The model under review builds one solid part; all positions refer to its coordinate system, in mm. A direction names the side the tool comes from. Coordinates: 2 decimals unless noted, no trailing zeros. Write each loop counter-clockwise with the first axis right and the second up, starting at its lowest first coordinate (ties: lowest second). Pieces come first, ordered by that corner, then holes. Notation, with made-up numbers: (49, 63.25) - (80, 63.25) arc R20 ccw to (80, 90.25) - close; hole circle Ø4 at (-35, -13). An arc over 180 degrees is marked (long way). Put each result on its own line as item: value.
from build123d import *

# Parameters (mm, degrees)
CROQUIS1_W              = 45.4
CROQUIS1_H              = 20.4
SALIENTE_EXTRUIR1_DEPTH = 1.6
CROQUIS2_R              = 0.7
CORTAR_EXTRUIR1_DEPTH   = 1
SALIENTE_EXTRUIR2_DEPTH = 0.5
SALIENTE_EXTRUIR3_DEPTH = 3
CROQUIS9_R              = 7.95
SALIENTE_EXTRUIR4_DEPTH = 11
CROQUIS10_W             = 10
CROQUIS10_H             = 1
SALIENTE_EXTRUIR5_DEPTH = 2
CROQUIS12_W             = 0.5
CROQUIS12_H             = 0.5
REDONDEO4_R             = 0.7
MATRIZL1_COUNT          = 4
MATRIZL1_PITCH          = 2.5
REDONDEO5_R             = 1
CROQUIS13_W             = 9
CROQUIS13_H             = 3
SALIENTE_EXTRUIR6_DEPTH = 1.5
MATRIZL2_COUNT          = 2
MATRIZL2_PITCH          = 18
CROQUIS14_W             = 3
CROQUIS14_H             = 9
SALIENTE_EXTRUIR7_DEPTH = 1.5
REDONDEO6_R             = 0.7


with BuildPart() as part:
    # Croquis1 → Saliente-Extruir1 (new body)
    with BuildSketch(Plane(origin=(0, 0, 0), x_dir=(1, 0, 0), z_dir=(0, 1, 0))):
        Rectangle(CROQUIS1_W, CROQUIS1_H)
    extrude(amount=SALIENTE_EXTRUIR1_DEPTH)

    # Croquis2 → Cortar-Extruir1 (cut)
    with BuildSketch(Plane(origin=(0, 1.6, 0), x_dir=(1, 0, 0), z_dir=(0, 1, 0))):
        with Locations((-21.5, 9)):
            Circle(CROQUIS2_R)
        with Locations((21.5, 9)):
            Circle(CROQUIS2_R)
        with Locations((21.5, -9)):
            Circle(CROQUIS2_R)
        with Locations((-21.5, -9)):
            Circle(CROQUIS2_R)
    extrude(amount=-CORTAR_EXTRUIR1_DEPTH, mode=Mode.SUBTRACT)

    # Croquis3 → Saliente-Extruir2 (add)
    with BuildSketch(Plane(origin=(0, 1.6, 0), x_dir=(1, 0, 0), z_dir=(0, 1, 0))):
        with BuildLine():
            Line((-4.202221616, 9.535810589), (4.202221616, 9.535810589))
            ThreePointArc((4.202221616, 9.535810589), (5.818460699, 7.919571506), (4.202221616, 6.303332424))
            Line((4.202221616, 6.303332424), (-4.202221616, 6.303332424))
            ThreePointArc((-4.202221616, 6.303332424), (-5.818460699, 7.919571506), (-4.202221616, 9.535810589))
        make_face()
        with BuildLine():
            Line((-4.202221616, 9.304919292), (4.202221616, 9.304919292))
            ThreePointArc((4.202221616, 9.304919292), (5.587569401, 7.919571506), (4.202221616, 6.534223721))
            Line((4.202221616, 6.534223721), (-4.202221616, 6.534223721))
            ThreePointArc((-4.202221616, 6.534223721), (-5.587569401, 7.919571506), (-4.202221616, 9.304919292))
        make_face(mode=Mode.SUBTRACT)
    extrude(amount=SALIENTE_EXTRUIR2_DEPTH)

    # Croquis8 → Saliente-Extruir3 (add)
    with BuildSketch(Plane(origin=(0, 1.6, 0), x_dir=(1, 0, 0), z_dir=(0, 1, 0))):
        with BuildLine():
            Line((-4.202221616, 9.304919292), (4.202221616, 9.304919292))
            ThreePointArc((4.202221616, 9.304919292), (5.587569401, 7.919571506), (4.202221616, 6.534223721))
            Line((4.202221616, 6.534223721), (-4.202221616, 6.534223721))
            ThreePointArc((-4.202221616, 6.534223721), (-5.587569401, 7.919571506), (-4.202221616, 9.304919292))
        make_face()
    extrude(amount=SALIENTE_EXTRUIR3_DEPTH)

    # Croquis9 → Saliente-Extruir4 (add)
    with BuildSketch(Plane(origin=(0, 1.6, 0), x_dir=(1, 0, 0), z_dir=(0, 1, 0))):
        with Locations((-13.1, 0)):
            Circle(CROQUIS9_R)
        with Locations((13.1, 0)):
            Circle(CROQUIS9_R)
    extrude(amount=SALIENTE_EXTRUIR4_DEPTH)

    # Croquis10 → Saliente-Extruir5 (add)
    with BuildSketch(Plane.XZ):
        with Locations((-0.012747973, 9.7)):
            Rectangle(CROQUIS10_W, CROQUIS10_H)
    extrude(amount=SALIENTE_EXTRUIR5_DEPTH)

    # Barrer1: sweep along a curve in space
    with BuildLine() as barrer1_path:
        Line((-3.762747973, -2, 9.7), (-3.762747973, -4, 9.7))
        Line((-3.762747973, -4, 9.7), (-3.762747973, -4, 16.7))
    # Croquis12 → Barrer1 (sweep)
    with BuildSketch(Plane.XZ.offset(2)):
        with Locations((-3.762747973, 9.7)):
            Rectangle(CROQUIS12_W, CROQUIS12_H)
    barrer1 = sweep(path=barrer1_path.line, transition=Transition.RIGHT)

    # Redondeo4
    redondeo4_edges = [part.edges().sort_by_distance(p)[0] for p in [
        (-3.762747973, -4.25, 9.45),
    ]]
    fillet(redondeo4_edges, radius=REDONDEO4_R)

    # MatrizL1: Barrer1 ×4
    with Locations(*[(i * MATRIZL1_PITCH, 0, 0) for i in range(1, MATRIZL1_COUNT)]):
        add(barrer1)

    # Redondeo5
    redondeo5_edges = [part.edges().sort_by_distance(p)[0] for p in [
        (-21.05, 12.6, 0),
        (5.15, 12.6, 0),
    ]]
    fillet(redondeo5_edges, radius=REDONDEO5_R)

    # Croquis13 → Saliente-Extruir6 (add)
    with BuildSketch(Plane.XZ):
        Rectangle(CROQUIS13_W, CROQUIS13_H)
    saliente_extruir6 = extrude(amount=SALIENTE_EXTRUIR6_DEPTH)

    # MatrizL2: Saliente-Extruir6 ×2
    with Locations(*[(i * MATRIZL2_PITCH, 0, 0) for i in range(1, MATRIZL2_COUNT)]):
        add(saliente_extruir6)

    # Croquis14 → Saliente-Extruir7 (add)
    with BuildSketch(Plane.XZ):
        with Locations((-19.2, -0.292211089)):
            Rectangle(CROQUIS14_W, CROQUIS14_H)
    extrude(amount=SALIENTE_EXTRUIR7_DEPTH)

    # Redondeo6
    redondeo6_edges = [part.edges().sort_by_distance(p)[0] for p in [
        (-1.262747973, -4.25, 9.45),
        (1.237252027, -4.25, 9.45),
        (3.737252027, -4.25, 9.45),
    ]]
    fillet(redondeo6_edges, radius=REDONDEO6_R)


solid = part.part
1. Consider section C-C on y = 10.5. State the section outline as (x, z) points, plus the area to 3 significant figures.
Determined:
outline: circle Ø15.9 at (-13.1, 0); circle Ø15.9 at (13.1, 0)
area: 397 mm^2
2. Consider section B-B on x = -13.1. State the section outline as (y, z) points.
Determined:
outline: (0, -10.2) - (1.6, -10.2) - (1.6, -7.95) - (11.6, -7.95) arc R1 ccw to (12.6, -6.95) - (12.6, 6.95) arc R1 ccw to (11.6, 7.95) - (1.6, 7.95) - (1.6, 10.2) - (0, 10.2) - close
3. Consider section A-A on z = 13.25. State the section outline as (x, y) points, plus the area to 4 significant figures.
Determined:
outline: (-4.01, -4.25) - (-3.51, -4.25) - (-3.51, -3.75) - (-4.01, -3.75) - close; (-1.51, -4.25) - (-1.01, -4.25) - (-1.01, -3.75) - (-1.51, -3.75) - close; (0.99, -4.25) - (1.49, -4.25) - (1.49, -3.75) - (0.99, -3.75) - close; (3.49, -4.25) - (3.99, -4.25) - (3.99, -3.75) - (3.49, -3.75) - close
area: 1.000 mm^2
4. Consider section D-D on z = 0. State the section outline as (x, y) points.
Determined:
outline: (-22.7, 0) - (-20.7, 0) - (-20.7, -1.5) - (-17.7, -1.5) - (-17.7, 0) - (-4.5, 0) - (-4.5, -1.5) - (4.5, -1.5) - (4.5, 0) - (13.5, 0) - (13.5, -1.5) - (22.5, -1.5) - (22.5, 0) - (22.7, 0) - (22.7, 1.6) - (21.05, 1.6) - (21.05, 11.6) arc R1 ccw to (20.05, 12.6) - (6.15, 12.6) arc R1 ccw to (5.15, 11.6) - (5.15, 1.6) - (-5.15, 1.6) - (-5.15, 11.6) arc R1 ccw to (-6.15, 12.6) - (-20.05, 12.6) arc R1 ccw to (-21.05, 11.6) - (-21.05, 1.6) - (-22.7, 1.6) - close
5. For pin 1 Ø4 at (x, y) = (-18, 5.5) entering from -Z; pin 2 Ø12 at (x, z) = (3.5, 12.5) entering from +Y; pin 3 Ø2.5 at (y, z) = (-3.5, 13.5) entering from -X, all flat-tipped, find the tip position at first contact; note any pin that passes through.
Determined:
pin 1: stops at z = -7.4
pin 2: stops at y = 1.6
pin 3: stops at x = -4.01
6. The part is to be moulded in two halves that separate along X. For faces 6 (the flat face through (0, 3, -6.534)), 7 (the flat face through (18, -1, 1.5)), 8 (the flat face through (-5.013, -1, 10)), say which applies: +X half, -X half, draft (parallel to the pull), parting line (faces both ways), or undercut.
Determined:
face 6: undercut
face 7: draft
face 8: -X half
7. To check wall thickness, follow probe 1 along Z at (x, y) = (-21.5, 1); probe 2 along X at (y, z) = (0.9, 9); probe 3 along Y at (x, z) = (1.5, -6). State the ranges of each line that lie inside material, in increasing order.
Determined:
probe 1: z = -10.2 to -9.7, -8.3 to 8.3, 9.7 to 10.2
probe 2: x = -22.7 to -22.2, -20.8 to 20.8, 22.2 to 22.7
probe 3: y = 0 to 1.6
8. Machinability: for faces 1 (the flat face through (18, -1, -1.5)), 2 (the flat face through (0, -1, 1.5)), 3 (the flat face through (-19, -1, 4.208)), 4 (the flat face through (-3.513, -4, 13)), 5 (the cylindrical face through (-5.818, 1.846, -7.884)), which of the approach directions +Z, -Z, +X, -X, +Y, -Y give a long, thin tool a straight path to every point of the face, cutting with its end or side? Answer none if there is none.
Determined:
face 1: -Z, +X, -Y
face 2: +X, -Y
face 3: +Z, +X, -X, -Y
face 4: +Z, -Z, -Y
face 5: +Y
